Autodesk Inventor part; units mm, degrees
ref_plane "YZ Plane" through (0, 0, 0) normal (1, 0, 0) x (0, 1, 0)
ref_plane "XZ Plane" through (0, 0, 0) normal (0, 1, 0) x (-1, 0, 0)
ref_plane "XY Plane" through (0, 0, 0) normal (0, 0, 1) x (1, 0, 0)
sketch "スケッチ1" plane through (0, 0, 0) normal (0, 0, 1) x (1, 0, 0)
  circle A0 centre (0, 0) radius 6
  dimension "d0" = 12
extrude "押し出し1" add sketch "スケッチ1" along normal blind 1
sketch "スケッチ2" plane through (0, 0, 1) normal (0, 0, 1) x (1, 0, 0)
  circle A0 centre (0, 0) radius 4
  circle A1 centre (0, 0) radius 3
  dimension "d3" = 8
  dimension "d4" = 6
extrude "押し出し2" add sketch "スケッチ2" along normal blind 1.5
hole "穴1" at (0, 0, 0) direction (0, 0, 1) diameter 6 end through all
properties part number "GFM-0608-025"
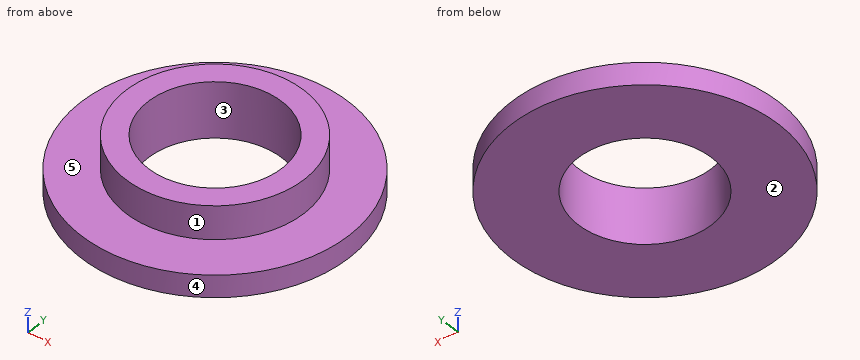
Work out the finished part from the listing and answer in its coordinate system (mm). Face numbers are marked on the shaded views. A direction names the side the tool comes from. Give positions to 0.01 mm unless a question says otherwise; leave off trailing zeros. Loops run counter-clockwise (first coordinate to the right, second up) from the corner with the lowest first, then second, coordinate; pieces in that order, holes last. Notation, with made-up numbers: (-5, -39) - (30, -39) arc R16 cw to (30, -27) - close; hole circle Ø4 at (83, 13). An arc over 180 degrees is marked (long way). Answer in a Markdown table with one row per item. Add a question column.
Q1. The part is cut by section A-A (y = 0). Determine the outline of the cut face in (x, z), and give its area (3 significant figures).
Q2. Determine the mould class of the marked faces 3, 4 and 5 for opening direction Y: released by +Y, released by -Y, zero draft, split by the parting line, or undercut.
Q3. This flat-tipped pin is pushed along its axis until it touches: P1, Ø1.5, axis at x = 1.5, z = 1, coming from the -Y side. Where does it stop, or does it pass through?
Q4. A tool of negligible diameter and unlimited length cuts with its end or side. For the marked faces 1 and 2, from which of +Z, -Z, +X, -X, +Y, -Y can it reach the whole face along a straight path? Write none if from no direction.
Q5. The part is cut by section D-D (z = 0.7). Determine the outline of the cut face in (x, y).
Q6. The part is cut by section C-C (z = 1.8). Determine the outline of the cut face in (x, y), and give its area (3 significant figures).
Q7. Consider line 1 along Y through (x, z) = (0, 2.05); line 2 along Y through (x, z) = (0, 0.75); line 3 along Z through (x, y) = (3.25, -3.75). Determine where each line is inside the solid, lowest interval first.
Solution:
| question | item | result |
|---|---|---|
| 1 | outline | (-6, 0) - (-3, 0) - (-3, 2.5) - (-4, 2.5) - (-4, 1) - (-6, 1) - close; (3, 0) - (6, 0) - (6, 1) - (4, 1) - (4, 2.5) - (3, 2.5) - close |
| 1 | area | 9.00 mm² |
| 2 | face 3 | undercut |
| 2 | face 4 | split by the parting line |
| 2 | face 5 | zero draft |
| 3 | P1 | stops at y = -5.95 |
| 4 | face 1 | +Z |
| 4 | face 2 | -Z, +X, -X, +Y, -Y |
| 5 | outline | circle Ø12 at (0, 0); hole circle Ø6 at (0, 0) |
| 6 | outline | circle Ø8 at (0, 0); hole circle Ø6 at (0, 0) |
| 6 | area | 22.0 mm² |
| 7 | line 1 | y = -4 to -3, 3 to 4 |
| 7 | line 2 | y = -6 to -3, 3 to 6 |
| 7 | line 3 | z = 0 to 1 |
